Autodesk Inventor part; units mm, degrees
ref_plane "YZ Plane" through (0, 0, 0) normal (1, 0, 0) x (0, 1, 0)
ref_plane "XZ Plane" through (0, 0, 0) normal (0, 1, 0) x (-1, 0, 0)
ref_plane "XY Plane" through (0, 0, 0) normal (0, 0, 1) x (1, 0, 0)
sketch "Sketch1" plane through (0, 0, 0) normal (1, 0, 0) x (0, 1, 0)
  line L0 (0, 0) -> (2.5, 0)
  line L1 (2.5, 0) -> (2.5, -12.642)
  line L2 (0, -15.6) -> (0, 0)
  arc A0 (0, -15.6) -> (2.5, -12.642) centre (3, -15.6) ccw
  circle A1 centre (3, -15.6) radius 1.6
  point P0 (2.5, -5.2)
  dimension "d0" = 3
  dimension "d1" = 3.2
  dimension "d2" = 2.5
  dimension "d3" = 5.2
  dimension "d4" = 10.4
  dimension "d5" = 3
extrude "Extrusion1" add sketch "Sketch1" along normal blind 43.5
sketch "Sketch2" plane through (0, 0, -15.6) normal (0, -1, 0) x (1, 0, 0)
  line L0 (0, -3) -> (43.5, -3)
  line L1 (26.875, -3) -> (16.625, -3)
  line L2 (16.625, -3) -> (16.625, 5)
  line L3 (16.625, 5) -> (26.875, 5)
  line L4 (26.875, 5) -> (26.875, -3)
  line L5 (43.5, -3) -> (43.5, 3)
  line L6 (43.5, -3) -> (36.5, -3)
  line L7 (36.5, -3) -> (36.5, 5)
  line L8 (36.5, 5) -> (43.5, 5)
  line L9 (43.5, 5) -> (43.5, -3)
  line L10 (0, -3) -> (7, -3)
  line L11 (7, -3) -> (7, 5)
  line L12 (7, 5) -> (0, 5)
  line L13 (0, 5) -> (0, -3)
  line L14 (43.5, 15.6) -> (43.5, 0)
  point P0 (0, 15.6)
  point P1 (43.5, 2.958)
  dimension "d8" = 10.25
  dimension "d9" = 43.5
  dimension "d10" = 16.625
  dimension "d11" = 8
  dimension "d12" = 7
  dimension "d13" = 7
extrude "Extrusion2" cut sketch "Sketch2" against normal through all
sketch "Sketch3" plane through (0, 2.5, 0) normal (0, 1, 0) x (1, 0, 0)
  line L0 (0, 5.2) -> (43.5, 5.2) construction
  line L1 (43.5, 10.6) -> (43.5, 0) construction
  point P0 (0, 0)
  point P1 (5.75, 5.2)
  point P2 (37.75, 5.2)
  dimension "d16" = 32
  dimension "d17" = 43.5
  dimension "d18" = 5.75
hole "Hole1" at (5.75, 2.5, -5.2) at (37.75, 2.5, -5.2) direction (0, -1, 0) diameter 3.4 depth 2.5 countersink diameter 6.3 countersink angle 90
fillet "Fillet1" radius 2 4 edges at (0, 1.25, -10.6) (43.5, 1.25, -10.6) (11.8125, 2.5, -12.642) (31.6875, 2.5, -12.642)
equation "\"d5\" = d0"
equation "\"d10\" = -0.5 * d8 + 0.5 * d9"
equation "\"d13\" = d12"
properties part number "hinge_v1"
Verification items for the finished model (mm, model axes). A direction names the side the tool comes from. Give positions to 0.01 mm unless a question says otherwise; leave off trailing zeros. Order: outer loops, then holes, each group sorted by start corner. A loop starts at its lowest first (then second) coordinate and runs counter-clockwise, first axis right, second up. Notation, with made-up numbers: M 44.5,34 L 58.5,34 A25 cw 58.5,71 Z; hole C -6,79 d11. An arc over 180 degrees is marked long. Answer in a Markdown table with one row per item. Add a question column.
Item 1: Gauge pin test, flat ends, axial feed: pin 1 (2.5 mm diameter, centred on y = 3, z = -15.6, fed in from -X); pin 2 (0.8 mm diameter, centred on x = 20, y = 1, fed in from -Z); pin 3 (3 mm diameter, centred on x = 28, z = -7, fed in from +Y); pin 4 (4.5 mm diameter, centred on x = 5.75, z = -5.2, fed in from +Y). Record the tip position at first contact, or that the pin passes through.
Item 2: Section check C-C, the plane z = -12. Enter the section's corners in (x, y) (3 decimals), and give its area (3 significant figures).
Item 3: Mould release check, pull along Z, two halves, no side actions. Record for faces 4 (the cylindrical face through (32, 3, -14)), 5 (the flat face through (21, 2.5, -5)), 6 (the cylindrical face through (31.75, 2.88, -12)): released by +Z, released by -Z, zero draft, split by the parting line, or undercut.
Item 4: Tool access check on faces 1 (the flat face through (36.5, 2, -14)), 2 (the flat face through (5, 1, -10.6)), 3 (the flat face through (22, 1, -10.6)). Record the directions out of +Z, -Z, +X, -X, +Y, -Y that give a thin tool (end or side, any length) a straight path to the whole face; none if there is none.
Item 5: Section check A-A, the plane x = 37.75. Enter the section's corners in (y, z), and give its area (3 significant figures).
Item 6: Scan lines: probe 1 along X at (y, z) = (2.45, -3); probe 2 along X at (y, z) = (0.45, -5.2); probe 3 along Z at (x, y) = (5.75, 0.35). Record each from-to range of solid material in increasing order. Write a range as from..to.
Item 7: Section check B-B, the plane z = -5.2. Enter the section's corners in (x, y), and give its area (3 significant figures).
Item 8: Section check D-D, the plane y = 0.45. Enter the section's corners in (x, z) (3 decimals), and give its area (3 significant figures).
Filled sheet:
| question | item | result |
|---|---|---|
| 1 | pin 1 | passes through |
| 1 | pin 2 | stops at z = -10.6 |
| 1 | pin 3 | stops at y = 2.5 |
| 1 | pin 4 | stops at y = 1.6 |
| 2 | outline | M 7,0 L 16.625,0 L 16.625,2.878 L 7,2.878 Z; M 26.875,0 L 36.5,0 L 36.5,2.878 L 26.875,2.878 Z |
| 2 | area | 55.4 mm^2 |
| 3 | face 4 | undercut |
| 3 | face 5 | zero draft |
| 3 | face 6 | released by +Z |
| 4 | face 1 | -Z, +X, +Y, -Y |
| 4 | face 2 | -Z, -X, +Y, -Y |
| 4 | face 3 | -Z, +Y, -Y |
| 5 | outline | M 0,-10.6 L 2.5,-10.6 L 2.5,-8.35 L 1.05,-6.9 L 0,-6.9 Z; M 0,-3.5 L 1.05,-3.5 L 2.5,-2.05 L 2.5,0 L 0,0 Z |
| 5 | area | 15.9 mm^2 |
| 6 | probe 1 | x = 0..3.57, 7.93..35.57, 39.93..43.5 |
| 6 | probe 2 | x = 0..4.05, 7.45..36.05, 39.45..43.5 |
| 6 | probe 3 | z = -10.6..-6.9, -3.5..0 |
| 7 | outline | M 0,0 L 4.05,0 L 4.05,1.05 L 2.6,2.5 L 0,2.5 Z; M 7.45,0 L 36.05,0 L 36.05,1.05 L 34.6,2.5 L 8.9,2.5 L 7.45,1.05 Z; M 39.45,0 L 43.5,0 L 43.5,2.5 L 40.9,2.5 L 39.45,1.05 Z |
| 7 | area | 87.5 mm^2 |
| 8 | outline | M 0,-8.6 A2 ccw 2,-10.6 L 7,-10.6 L 7,-17.18 L 16.625,-17.18 L 16.625,-10.6 L 26.875,-10.6 L 26.875,-17.18 L 36.5,-17.18 L 36.5,-10.6 L 41.5,-10.6 A2 ccw 43.5,-8.6 L 43.5,0 L 0,0 Z; hole C 5.75,-5.2 d3.4; hole C 37.75,-5.2 d3.4 |
| 8 | area | 568 mm^2 |
